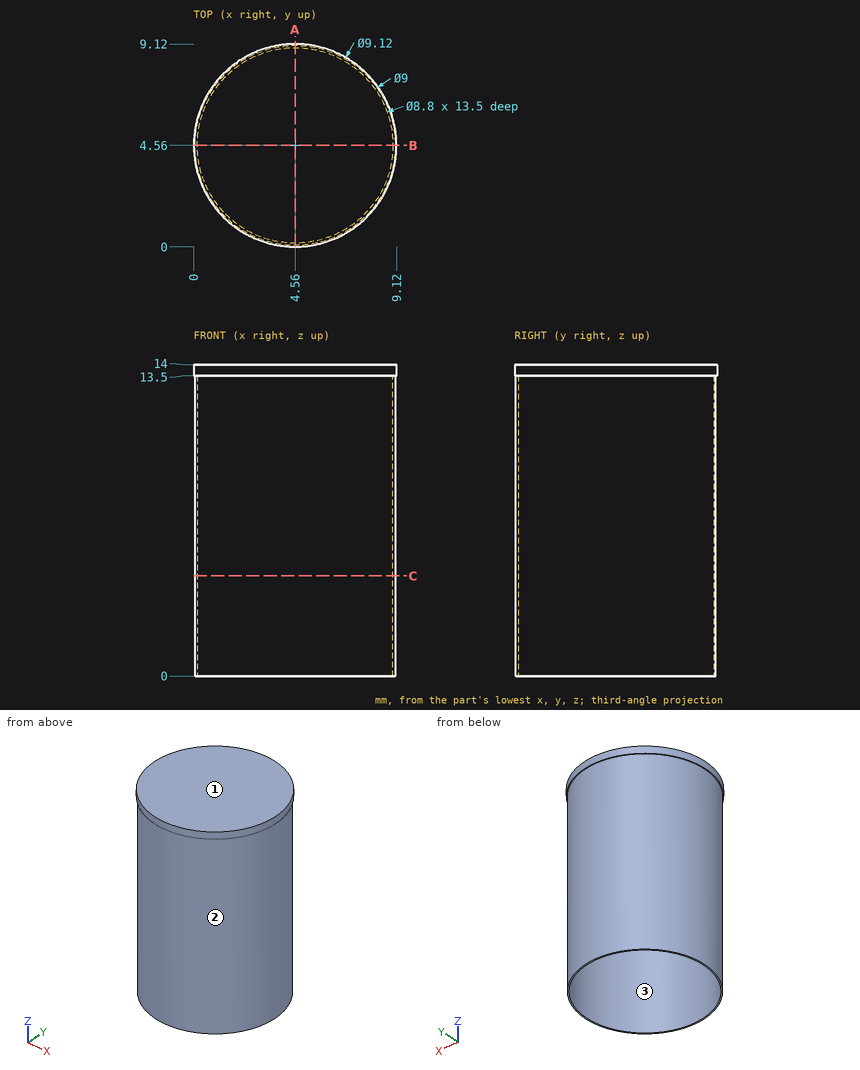
Design review of the part shown in the three views and the two pictorial views. Dimensions are in mm from the part's minimum x, y and z. Round coordinates to 2 decimals unless told otherwise and drop trailing zeros. Loops run counter-clockwise (first coordinate to the right, second up) from the corner with the lowest first, then second, coordinate; pieces in that order, holes last. Notation, with made-up numbers: M 63.25,-13.75 L 95.25,-13.75 A17 cw 95.25,2.25 Z; hole C 9,-34.75 d11. An arc over 180 degrees is marked long. Answer as a JSON object with one key per item and string values.
Item 1: The part is to be moulded in two halves that separate along Y. For the marked faces 1, 2 and 3, say which applies: +Y half, -Y half, draft (parallel to the pull), parting line (faces both ways), or undercut.
Check sheet entries:
{"face 1": "draft", "face 2": "parting line", "face 3": "undercut"}
Item 2: For line 1 along Z through (x, y) = (5.75, 7.25); line 2 along Y through (x, z) = (8, 9.5); line 3 along Y through (x, z) = (8.5, 3.75), list the stretches that pass through material, from the lowest coordinate up.
Check sheet entries:
{"line 1": "13.5 to 14", "line 2": "1.66 to 1.82, 7.3 to 7.46", "line 3": "2.39 to 2.6, 6.52 to 6.73"}
Item 3: Clearance check with flat-ended pins moving along their axes: P1, Ø4, axis at y = 2, z = 8, coming from the -X side (3 decimals); P2, Ø1.5, axis at x = 5.5, z = 3, coming from the -Y side; P3, Ø2.5, axis at x = 6, y = 6, coming from the -Z side. State where each tip first meets the part, or that it passes through.
Check sheet entries:
{"P1": "x = 0.095", "P2": "y = 0.06", "P3": "z = 13.5"}
Item 4: We need section A-A, the plane x = 4.56. State the section outline as (y, z) points, and give its area (3 significant figures).
Check sheet entries:
{"outline": "M 0,13.5 L 0.06,13.5 L 0.06,0 L 0.16,0 L 0.16,13.5 L 8.96,13.5 L 8.96,0 L 9.06,0 L 9.06,13.5 L 9.12,13.5 L 9.12,14 L 0,14 Z", "area": "7.26 mm2"}
Item 5: We need section C-C, the plane z = 4.5. State the section outline as (x, y) points.
Check sheet entries:
{"outline": "C 4.56,4.56 d9; hole C 4.56,4.56 d8.8"}
